Geometry: final body of the model. Coordinates: model frame, mm. Face numbers are marked on the shaded views. A direction names the side the tool comes from. Give positions to 0.01 mm unless a question says otherwise; leave off trailing zeros. Write each loop counter-clockwise with the first axis right and the second up, starting at its lowest first coordinate (ties: lowest second). Pieces come first, ordered by that corner, then holes. Notation, with made-up numbers: (-15, -21) -> (34, -21) arc R17 ccw to (34, 6) -> close; hole circle Ø8 at (40, 12). An arc over 180 degrees is marked (long way). Use CSV: the item, a comma, the result in double quotes. Start each with the question number.
1) Section A-A (x = -17). Count the separate pieces of the cut face and the enclosed holes in it, plus the area to 3 significant figures.
2) Section C-C (x = 16.5). Output: boundary loops of the cut face in (y, z), plus the area to 3 significant figures.
3) Section B-B (y = -27). Output: boundary loops of the cut face in (x, z).
4) Contact query for flat-ended pins moving along their axis: P1, Ø3, axis at x = 26, y = 35, coming from the +Z side; P2, Ø1.5, axis at x = 11.5, y = -20.5, coming from the -Z side. Output: stop coordinate, or through.
5) Material intervals for line 1 (Y direction, x = 26, z = 7.25); line 2 (Y direction, x = 25, z = 20.25); line 3 (X direction, y = 4.5, z = 8.5), sorted ascending. Write a range as [from, to].
6) Set-up query: the marked faces 5 and 6. Return all of +Z, -Z, +X, -X, +Y, -Y with unobstructed straight access to the full face (end or side cutting, diameter ignored); none if empty.
7) Draft query along X for the marked faces 1, 2, 3 and 4. Return one class per face: pulls with the +X half, pulls with the -X half, needs draft (parallel to the pull), parting line crosses it, or undercut.
```python
from build123d import *

# Parameters (mm, degrees)
SKETCH024_W     = 62
SKETCH024_H     = 84
PAD007_DEPTH    = 23
SKETCH025_W     = 50.4
SKETCH025_H     = 80.4
POCKET015_DEPTH = 21
SKETCH026_W     = 10
SKETCH026_H     = 10
PAD008_DEPTH    = 19.2
SKETCH027_R     = 1.7
POCKET016_DEPTH = 21.2
POCKET017_DEPTH = 18.4
FILLET004_R     = 2


with BuildPart() as part:
    # Sketch024 → Pad007 (new body)
    with BuildSketch(Plane.XY):
        Rectangle(SKETCH024_W, SKETCH024_H)
    extrude(amount=PAD007_DEPTH)

    # Sketch025 (on Face6 of Pad007) → Pocket015 (cut)
    with BuildSketch(Plane.XY.offset(23)):
        with Locations((4, 0)):
            Rectangle(SKETCH025_W, SKETCH025_H)
    extrude(amount=-POCKET015_DEPTH, mode=Mode.SUBTRACT)

    # Sketch026 (on Face11 of Pocket015) → Pad008 (join)
    with BuildSketch(Plane.XY.offset(2)):
        with Locations((-16.2, 35.2)):
            Rectangle(SKETCH026_W, SKETCH026_H)
        with Locations((24.2, 35.2)):
            Rectangle(SKETCH026_W, SKETCH026_H)
        with Locations((24.2, -35.2)):
            Rectangle(SKETCH026_W, SKETCH026_H)
        with Locations((-16.2, -35.2)):
            Rectangle(SKETCH026_W, SKETCH026_H)
    extrude(amount=PAD008_DEPTH)

    # Sketch027 (on Face19 of Pad008) → Pocket016 (cut)
    with BuildSketch(Plane.XY.offset(21.2)):
        with Locations((25, 36)):
            Circle(SKETCH027_R)
        with Locations((-17, 36)):
            Circle(SKETCH027_R)
        with Locations((25, -36)):
            Circle(SKETCH027_R)
        with Locations((-17, -36)):
            Circle(SKETCH027_R)
    extrude(amount=-POCKET016_DEPTH, mode=Mode.SUBTRACT)

    # Sketch028 (on Face4 of Pocket016) → Pocket017 (cut)
    with BuildSketch(Plane(origin=(0, 0, 0), x_dir=(1, 0, 0), z_dir=(0, 0, -1))):
        Polygon((-15.412287, 33.25), (-13.824574, 36), (-15.412287, 38.75), (-18.587713, 38.75), (-20.175426, 36), (-18.587713, 33.25), align=None)
        Polygon((23.412287, 33.25), (26.587713, 33.25), (28.175426, 36), (26.587713, 38.75), (23.412287, 38.75), (21.824574, 36), align=None)
        Polygon((-15.412287, -33.25), (-18.587713, -33.25), (-20.175426, -36), (-18.587713, -38.75), (-15.412287, -38.75), (-13.824574, -36), align=None)
        Polygon((26.587713, -33.25), (23.412287, -33.25), (21.824574, -36), (23.412287, -38.75), (26.587713, -38.75), (28.175426, -36), align=None)
    extrude(amount=-POCKET017_DEPTH, mode=Mode.SUBTRACT)

    # Fillet004
    fillet004_edges = [part.edges().sort_by_distance(p)[0] for p in [
        (-31, -42, 11.5),
        (31, -42, 11.5),
        (31, 42, 11.5),
        (31, 0, 0),
        (0, -42, 0),
        (0, 42, 0),
        (-31, 42, 11.5),
        (-31, 0, 0),
    ]]
    fillet(fillet004_edges, radius=FILLET004_R)


solid = part.part
```
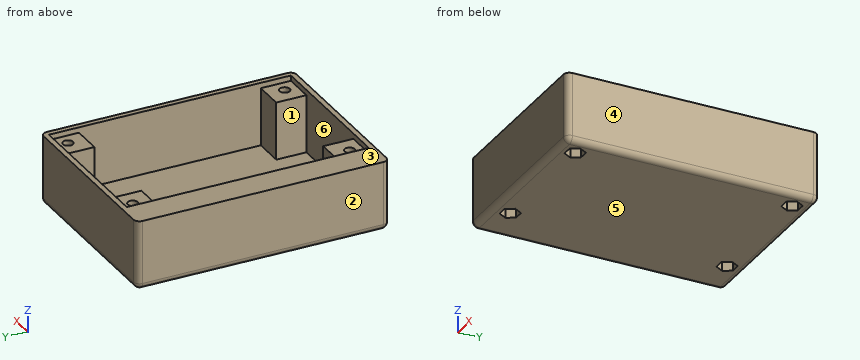
Answers follow:
1,separate pieces,"3"
1,enclosed holes,"0"
1,area,"404 mm^2"
2,outline,"(-42, 2) arc R2 ccw to (-40, 0) -> (40, 0) arc R2 ccw to (42, 2) -> (42, 23) -> (40.2, 23) -> (40.2, 2) -> (-40.2, 2) -> (-40.2, 23) -> (-42, 23) -> close"
2,area,"242 mm^2"
3,outline,"(-31, 2) arc R2 ccw to (-29, 0) -> (29, 0) arc R2 ccw to (31, 2) -> (31, 23) -> (29.2, 23) -> (29.2, 2) -> (-21.2, 2) -> (-21.2, 23) -> (-31, 23) -> close"
4,P1,"stops at z = 21.2"
4,P2,"stops at z = 0"
5,line 1,"y = [-42, -38.75], [-33.25, -30.2], [30.2, 33.25], [38.75, 42]"
5,line 2,"y = [-42, -37.7], [-34.3, -30.2], [30.2, 34.3], [37.7, 42]"
5,line 3,"x = [-31, -21.2], [29.2, 31]"
6,face 5,"-Z, +X, -X, +Y, -Y"
6,face 6,"+Z"
7,face 1,"undercut"
7,face 2,"pulls with the -X half"
7,face 3,"needs draft"
7,face 4,"pulls with the +X half"
